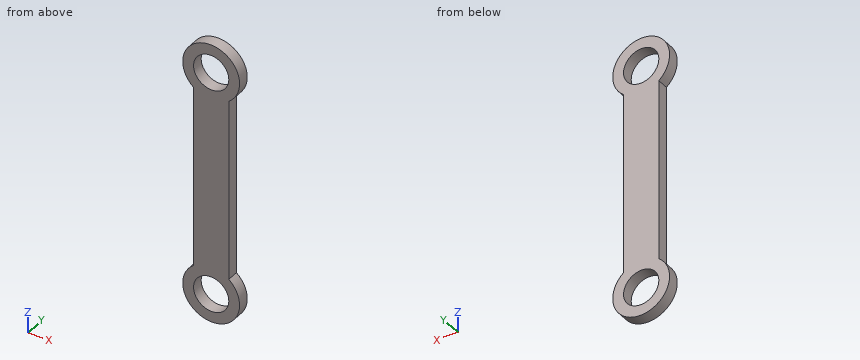
from build123d import *

# Parameters (mm, degrees)
F0_R          = 1.55
F1_DEPTH      = 4.5
F2_W          = 2.5
F2_H          = 6.339147
F3_DEPTH      = 4.051
F3_DEPTH_BACK = 0.951
F4_W          = 15.761445
F4_H          = 34.727139
F4_R          = 1.55
F5_DEPTH      = 3.5


with BuildPart() as f1:
    # F0 (on Front) → F1 (new body)
    with BuildSketch(Plane.XZ):
        with BuildLine():
            Line((14.506739, 11.988214), (14.506739, 28.065205))
            ThreePointArc((14.506739, 28.065205), (12.956739, 32.52671), (11.406739, 28.065205))
            Line((11.406739, 28.065205), (11.406739, 11.988214))
            ThreePointArc((11.406739, 11.988214), (12.956739, 7.52671), (14.506739, 11.988214))
        make_face()
        with Locations((12.956739, 10.02671)):
            Circle(F0_R, mode=Mode.SUBTRACT)
        with Locations((12.956739, 30.02671)):
            Circle(F0_R, mode=Mode.SUBTRACT)
    extrude(amount=F1_DEPTH)

    # F2 (on face) → F3 (cut, two sides)
    with BuildSketch(Plane.YZ.offset(14.506739)) as f3_sk:
        with Locations((-2.25, 30.034779)):
            Rectangle(F2_W, F2_H)
    extrude(amount=-F3_DEPTH, mode=Mode.SUBTRACT)
    extrude(f3_sk.sketch, amount=-F3_DEPTH_BACK, mode=Mode.SUBTRACT)

    # F4 (on face) → F5 (cut)
    with BuildSketch(Plane.XZ.offset(4.5)):
        with Locations((14.291149, 18.705026)):
            Rectangle(F4_W, F4_H)
        with BuildLine():
            ThreePointArc((14.506739, 11.988214), (12.956739, 7.52671), (11.406739, 11.988214))
            Line((11.406739, 11.988214), (11.406739, 28.065205))
            ThreePointArc((11.406739, 28.065205), (12.956739, 32.52671), (14.506739, 28.065205))
            Line((14.506739, 28.065205), (14.506739, 11.988214))
        make_face(mode=Mode.SUBTRACT)
        with BuildLine():
            Line((11.406739, 28.065205), (11.406739, 11.988214))
            ThreePointArc((11.406739, 11.988214), (12.956739, 7.52671), (14.506739, 11.988214))
            Line((14.506739, 11.988214), (14.506739, 28.065205))
            ThreePointArc((14.506739, 28.065205), (12.956739, 32.52671), (11.406739, 28.065205))
        make_face()
        with Locations((12.956739, 10.02671)):
            Circle(F4_R, mode=Mode.SUBTRACT)
        with Locations((12.956739, 30.02671)):
            Circle(F4_R, mode=Mode.SUBTRACT)
    extrude(amount=-F5_DEPTH, mode=Mode.SUBTRACT)


solid = f1.part
Model file for the job. Use its own axes, mm. Round coordinates to 2 decimals unless told otherwise and drop trailing zeros. Order: outer loops, then holes, each group sorted by start corner. A loop starts at its lowest first (then second) coordinate and runs counter-clockwise, first axis right, second up.
(1) Drill centre lines: line 1 (Z direction, x = 14.35, y = -0.8); line 2 (Z direction, x = 13.4, y = -0.05); line 3 (X direction, y = -0.75, z = 10). Where is each one in solid material? Low to high.
(2) Band-saw the part on C-C (x = 14.8). List the corners of the cut face in (y, z).
(3) Band-saw the part on B-B (z = 29.75). List the corners of the cut face in (x, y), then the cut area to 3 significant figures.
(4) Band-saw the part on A-A (x = 12.6). List the corners of the cut face in (y, z), then the cut area to 3 significant figures.
(5) Band-saw the part on D-D (y = -0.35). List the corners of the cut face in (x, z).
Verdict:
1. line 1: z = 7.95 to 9.35, 10.71 to 29.35, 30.71 to 32.1
1. line 2: z = 7.57 to 8.54, 11.51 to 28.54, 31.51 to 32.49
1. line 3: x = 10.46 to 11.41, 14.51 to 15.46
2. outline: (-1, 8.34) - (0, 8.34) - (0, 11.72) - (-1, 11.72) - close; (-1, 28.34) - (0, 28.34) - (0, 31.72) - (-1, 31.72) - close
3. outline: (10.47, -1) - (11.43, -1) - (11.43, 0) - (10.47, 0) - close; (14.48, -1) - (15.44, -1) - (15.44, 0) - (14.48, 0) - close
3. area: 1.92 mm2
4. outline: (-1, 7.55) - (0, 7.55) - (0, 8.52) - (-1, 8.52) - close; (-1, 11.54) - (0, 11.54) - (0, 28.52) - (-1, 28.52) - close; (-1, 31.54) - (0, 31.54) - (0, 32.5) - (-1, 32.5) - close
4. area: 18.9 mm2
5. outline: (11.41, 11.99) arc R2.5 ccw (long way) to (14.51, 11.99) - (14.51, 28.07) arc R2.5 ccw (long way) to (11.41, 28.07) - close; hole circle Ø3.1 at (12.96, 10.03); hole circle Ø3.1 at (12.96, 30.03)
